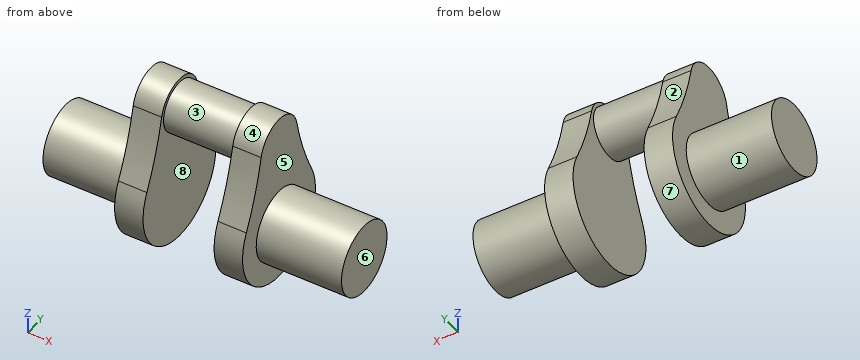
Autodesk Inventor part; units mm, degrees
ref_plane "Work Plane2" through (-25, 0, 60) normal (-1, 0, 0) x (0, 0, 1)
ref_plane "YZ Plane" through (0, 0, 0) normal (1, 0, 0) x (0, 1, 0)
ref_plane "XZ Plane" through (0, 0, 0) normal (0, 1, 0) x (-1, 0, 0)
sketch "Sketch4" plane through (0, 0, 0) normal (1, 0, 0) x (0, 1, 0)
  arc A0 (-35.8323, 17.7778) -> (35.8323, 17.7778) centre (0, 0) ccw
  arc A1 (19.5449, 64.2424) -> (-19.5449, 64.2424) centre (0, 60) ccw
  arc A2 (-35.8323, 17.7778) -> (-19.5449, 64.2424) centre (-214.9935, 106.6667) ccw
  arc A3 (19.5449, 64.2424) -> (35.8323, 17.7778) centre (214.9935, 106.6667) ccw
  dimension "d13" = 80
  dimension "d14" = 40
  dimension "d15" = 60
  dimension "d16" = 200
  dimension "d17" = 200
extrude "Extrusion4" add sketch "Sketch4" along normal blind 20
sketch "Sketch5" plane through (20, 0, 0) normal (1, 0, 0) x (0, 0, -1)
  arc A0 (-17.7778, -35.8323) -> (-17.7778, 35.8323) centre (0, 0) ccw
  circle A1 centre (0, 0) radius 25
  dimension "d20" = 50
extrude "Extrusion5" add sketch "Sketch5" along normal blind 60
sketch "Sketch6" plane through (0, 0, 0) normal (-1, 0, 0) x (0, 0, 1)
  arc A0 (64.2424, -19.5449) -> (64.2424, 19.5449) centre (60, 0) ccw
  circle A1 centre (60, 0) radius 17.5
  dimension "d23" = 35
extrude "Extrusion6" add sketch "Sketch6" along normal blind 50
ref_plane "Work Plane2" through (-25, 0, 60) normal (-1, 0, 0) x (0, 0, 1)
mirror "Mirror3" about plane through (-25, 0, 60) normal (-1, 0, 0) of "Extrusion4"
mirror "Mirror4" about plane through (-25, 0, 60) normal (-1, 0, 0) of "Extrusion5"
properties part number "crankshaft" material "Silicon Nitride"
For this review, take the finished solid that the model builds, in its own axes (mm). Face numbers are marked on the shaded views. A direction names the side the tool comes from. Round coordinates to 2 decimals unless told otherwise and drop trailing zeros. Order: outer loops, then holes, each group sorted by start corner. A loop starts at its lowest first (then second) coordinate and runs counter-clockwise, first axis right, second up.
Q1. We need section A-A, the plane z = 0. Give the boundary of the cut face in (x, y).
Findings below:
outline: (-130, -25) - (-70, -25) - (-70, -40) - (-50, -40) - (-50, 40) - (-70, 40) - (-70, 25) - (-130, 25) - close; (0, -40) - (20, -40) - (20, -25) - (80, -25) - (80, 25) - (20, 25) - (20, 40) - (0, 40) - close
Q2. We need section C-C, the plane y = -28.5. Give the boundary of the cut face in (x, z), plus the area to 3 significant figures.
Findings below:
outline: (-70, -28.07) - (-50, -28.07) - (-50, 34.42) - (-70, 34.42) - close; (0, -28.07) - (20, -28.07) - (20, 34.42) - (0, 34.42) - close
area: 2,500 mm2
Q3. We need section D-D, the plane x = -111.5. Give the boundary of the cut face in (y, z).
Findings below:
outline: circle Ø50 at (0, 0)
Q4. Insertion check: P1, Ø1.5, axis at y = 2, z = 27.5, coming from the +X side; P2, Ø5, axis at x = -87, y = -9, coming from the +Z side; P3, Ø8, axis at x = -26.5, y = 1.5, coming from the +Z side. Each pin has a flat end and moves straight along its axis. Give the tip position at first contact, or say it passes through.
Findings below:
P1: stops at x = 20
P2: stops at z = 24.14
P3: stops at z = 77.5
Q5. Wall thickness on line 1 (X direction, y = -13, z = 28.5); line 2 (X direction, y = -15.5, z = -12.5); line 3 (X direction, y = 2, z = 52.5): over which ranges is each line inside the solid? List them lowest first.
Findings below:
line 1: x = -70 to -50, 0 to 20
line 2: x = -130 to -50, 0 to 80
line 3: x = -70 to 20
Q6. Mouldability with a two-part tool opening along X and no side actions: class the marked faces 6, 7 and 8 as pulls with the +X half, pulls with the -X half, needs draft (parallel to the pull), parting line crosses it, or undercut.
Findings below:
face 6: pulls with the +X half
face 7: needs draft
face 8: undercut
Q7. Machinability: for the marked faces 1, 2, 3, 4 and 5, which of the approach directions +Z, -Z, +X, -X, +Y, -Y give a long, thin tool a straight path to every point of the face, cutting with its end or side? Answer none if there is none.
Findings below:
face 1: -X
face 2: +Z, +X, -X, +Y
face 3: none
face 4: +Z, +X, -X
face 5: +X
Q8. We need section B-B, the plane y = 0. Give the boundary of the cut face in (x, z), plus the area to 4 significant figures.
Findings below:
outline: (-130, -25) - (-70, -25) - (-70, -40) - (-50, -40) - (-50, 42.5) - (0, 42.5) - (0, -40) - (20, -40) - (20, -25) - (80, -25) - (80, 25) - (20, 25) - (20, 80) - (0, 80) - (0, 77.5) - (-50, 77.5) - (-50, 80) - (-70, 80) - (-70, 25) - (-130, 25) - close
area: 12,550 mm2
